from build123d import *

# Parameters (mm, degrees)
SKETCH_W        = 50
SKETCH_H        = 40
SKETCH_R        = 2.2
PAD_DEPTH       = 3
SKETCH001_W     = 50
SKETCH001_H     = 14
PAD001_DEPTH    = 60
POCKET_DEPTH    = 50
POCKET001_DEPTH = 14
FILLET_R        = 5
FILLET001_R     = 2
FILLET002_R     = 5


with BuildPart() as part:
    # Sketch → Pad (new body)
    with BuildSketch(Plane.XY):
        Rectangle(SKETCH_W, SKETCH_H)
        with Locations((-20, -15)):
            Circle(SKETCH_R, mode=Mode.SUBTRACT)
        with Locations((20, 15)):
            Circle(SKETCH_R, mode=Mode.SUBTRACT)
        with Locations((20, -15)):
            Circle(SKETCH_R, mode=Mode.SUBTRACT)
        with Locations((-20, 15)):
            Circle(SKETCH_R, mode=Mode.SUBTRACT)
    extrude(amount=PAD_DEPTH)

    # Sketch001 (on Face10 of Pad) → Pad001 (join)
    with BuildSketch(Plane.XY.offset(3)):
        Rectangle(SKETCH001_W, SKETCH001_H)
    extrude(amount=PAD001_DEPTH)

    # Sketch002 (on Face9 of Pad001) → Pocket (cut)
    with BuildSketch(Plane.YZ.offset(25)):
        Polygon((-2, 63), (-2, 58), (-4, 58), (-4, 18), (4, 18), (4, 58), (2, 58), (2, 63), align=None)
    extrude(amount=-POCKET_DEPTH, mode=Mode.SUBTRACT)

    # Sketch003 (on Face15 of Pocket) → Pocket001 (cut)
    with BuildSketch(Plane.XZ.offset(7)):
        Polygon((-10, 63), (0, 3), (25, 3), (25, 63), align=None)
    extrude(amount=-POCKET001_DEPTH, mode=Mode.SUBTRACT)

    # Fillet
    fillet_edges = [part.edges().sort_by_distance(p)[0] for p in [
        (-25, -20, 1.5),
        (25, -20, 1.5),
        (25, 20, 1.5),
        (-25, 20, 1.5),
    ]]
    fillet(fillet_edges, radius=FILLET_R)

    # Fillet001
    fillet001_edges = [part.edges().sort_by_distance(p)[0] for p in [
        (-10, -4.5, 63),
        (-25, -4.5, 63),
        (-10, 4.5, 63),
        (-25, 4.5, 63),
    ]]
    fillet(fillet001_edges, radius=FILLET001_R)

    # Fillet002
    fillet002_edges = [part.edges().sort_by_distance(p)[0] for p in [
        (-2.5, 0, 18),
        (-25, 0, 18),
    ]]
    fillet(fillet002_edges, radius=FILLET002_R)


solid = part.part
The model under review builds one solid part; all positions refer to its coordinate system, in mm. A direction names the side the tool comes from. Give positions to 0.01 mm unless a question says otherwise; leave off trailing zeros. Order: outer loops, then holes, each group sorted by start corner. A loop starts at its lowest first (then second) coordinate and runs counter-clockwise, first axis right, second up. Notation, with made-up numbers: M 65,41 L 124,41 A20 ccw 124,54 Z; hole C 30,-12 d11. An arc over 180 degrees is marked long. One line per question, with ' | ' between items. Start each with the question number.
1) Consider section C-C, the plane z = 40. Give the boundary of the cut face in (x, y), then the cut area to 3 significant figures.
2) Mouldability with a two-part tool opening along Y and no side actions: class faces 1 (the face through (-16, -4, 36)), 2 (the face through (-15, -7, 33)), 3 (the face through (-10.42, -4.46, 62.54)) as pulls with the +Y half, pulls with the -Y half, needs draft (parallel to the pull), parting line crosses it, or undercut.
3) Consider section D-D, the plane x = 3.5. Give the boundary of the cut face in (y, z), then the cut area to 3 significant figures.
4) Clearance check with flat-ended pins moving along their axes: P1, Ø5, axis at x = -14, z = 48, coming from the -Y side; P2, Ø6, axis at x = -17, y = 12, coming from the +Z side; P3, Ø18.5, axis at x = -12, z = 30.5, coming from the +Y side. State where each tip first meets the part, or that it passes through.
5) Consider section A-A, the plane z = 24. Give the boundary of the cut face in (x, y).
6) Consider section B-B, the plane x = -6. Give the boundary of the cut face in (y, z), then the cut area to 3 significant figures.
7) For faces 4 (the face through (-24, 0, 16)), 5 (the face through (5, 0, 3)), 6 (the face through (-17, 2, 60)), list the 3-axis set-ups (+Z, -Z, +X, -X, +Y, -Y) from which the entire face can be reached by the end or side of a thin tool; tool diameter is ignored.
8) Wall thickness on L1, parallel to Y at x = -20, z = 0.85; L2, parallel to Y at x = -19, z = 37.5; L3, parallel to Z at x = 3.5, y = 11: over which ranges is each line inside the solid? List them lowest first. Write a range as from..to.
Found:
1) outline: M -25,-7 L -6.17,-7 L -6.17,-4 L -25,-4 Z; M -25,4 L -6.17,4 L -6.17,7 L -25,7 Z | area: 113 mm²
2) face 1: undercut | face 2: pulls with the -Y half | face 3: needs draft
3) outline: M -20,0 L 20,0 L 20,3 L -20,3 Z | area: 120 mm²
4) P1: stops at y = -7 | P2: stops at z = 3 | P3: stops at y = 7
5) outline: M -25,-7 L -3.5,-7 L -3.5,-4 L -25,-4 Z; M -25,4 L -3.5,4 L -3.5,7 L -25,7 Z
6) outline: M -20,0 L 20,0 L 20,3 L 7,3 L 7,39 L 4,39 L 4,17.95 L -4,17.95 L -4,39 L -7,39 L -7,3 L -20,3 Z | area: 456 mm²
7) face 4: -X | face 5: +Z, +X | face 6: +Z, +X, -X
8) L1: y = -20..-17.2, -12.8..12.8, 17.2..20 | L2: y = -7..-4, 4..7 | L3: z = 0..3
